from build123d import *

# Parameters (mm, degrees)
SKETCH1_R           = 4.25
BOSS_EXTRUDE1_DEPTH = 9.6
BOSS_EXTRUDE2_DEPTH = 3.3
SKETCH3_OUTSIDE_W   = 42.178
SKETCH3_OUTSIDE_H   = 40.63
SKETCH3_OUTSIDE_R   = 4.25
CUT_EXTRUDE4_DEPTH  = 3.3
CUT_EXTRUDE4_TAPER  = 75
SKETCH5_OUTSIDE_W   = 42.178
SKETCH5_OUTSIDE_H   = 40.63
SKETCH5_OUTSIDE_R   = 4.25
CUT_EXTRUDE5_DEPTH  = 3.3
CUT_EXTRUDE5_TAPER  = 75
SKETCH6_R           = 2.9
BOSS_EXTRUDE3_DEPTH = 3
SKETCH7_R           = 3.95
BOSS_EXTRUDE4_DEPTH = 7.5
SKETCH8_R           = 1.5
CUT_EXTRUDE6_DEPTH  = 24.4
SKETCH9_R           = 2.25
CUT_EXTRUDE7_DEPTH  = 10
FILLET1_R           = 0.5
SKETCH10_R          = 1.5
CUT_EXTRUDE8_DEPTH  = 6.0000001
CHAMFER1_SIZE       = 1


with BuildPart() as part:
    # Sketch1 → Boss-Extrude1 (new body)
    with BuildSketch(Plane(origin=(0, 0, 0), x_dir=(1, 0, 0), z_dir=(0, 1, 0))):
        Circle(SKETCH1_R)
    extrude(amount=BOSS_EXTRUDE1_DEPTH)

    # Sketch2 → Boss-Extrude2 (add)
    with BuildSketch(Plane.XZ):
        Polygon((-2.886751346, 5), (-5.773502692, 0), (-2.886751346, -5), (2.886751346, -5), (5.773502692, 0), (2.886751346, 5), align=None)
    extrude(amount=BOSS_EXTRUDE2_DEPTH)

    # Sketch3 outside → Cut-Extrude4 (cut)
    with BuildSketch(Plane.XZ.offset(3.3)):
        Rectangle(SKETCH3_OUTSIDE_W, SKETCH3_OUTSIDE_H)
        Circle(SKETCH3_OUTSIDE_R, mode=Mode.SUBTRACT)
    extrude(amount=-CUT_EXTRUDE4_DEPTH, taper=CUT_EXTRUDE4_TAPER, mode=Mode.SUBTRACT)

    # Sketch5 outside → Cut-Extrude5 (cut)
    with BuildSketch(Plane(origin=(0, 0, 0), x_dir=(1, 0, 0), z_dir=(0, 1, 0))):
        Rectangle(SKETCH5_OUTSIDE_W, SKETCH5_OUTSIDE_H)
        Circle(SKETCH5_OUTSIDE_R, mode=Mode.SUBTRACT)
    extrude(amount=-CUT_EXTRUDE5_DEPTH, taper=CUT_EXTRUDE5_TAPER, mode=Mode.SUBTRACT)

    # Sketch6 → Boss-Extrude3 (add)
    with BuildSketch(Plane.XZ.offset(3.3)):
        Circle(SKETCH6_R)
    extrude(amount=BOSS_EXTRUDE3_DEPTH)

    # Sketch7 → Boss-Extrude4 (add)
    with BuildSketch(Plane.XZ.offset(6.3)):
        Circle(SKETCH7_R)
    extrude(amount=BOSS_EXTRUDE4_DEPTH)

    # Sketch8 → Cut-Extrude6 (cut, through all)
    with BuildSketch(Plane.XZ.offset(13.8)):
        Circle(SKETCH8_R)
    extrude(amount=-CUT_EXTRUDE6_DEPTH, mode=Mode.SUBTRACT)

    # Sketch9 → Cut-Extrude7 (cut)
    with BuildSketch(Plane.XZ.offset(13.8)):
        Circle(SKETCH9_R)
    extrude(amount=-CUT_EXTRUDE7_DEPTH, mode=Mode.SUBTRACT)

    # Fillet1
    fillet1_edges = [part.edges().sort_by_distance(p)[0] for p in [
        (-4.25, 0, 0),
        (-2.9, -3.3, 0),
        (-2.9, -6.3, 0),
    ]]
    fillet(fillet1_edges, radius=FILLET1_R)

    # Sketch10 → Cut-Extrude8 (cut, through all)
    with BuildSketch(Plane.XY):
        with Locations((0, 5.6)):
            Circle(SKETCH10_R)
    extrude(amount=-CUT_EXTRUDE8_DEPTH, mode=Mode.SUBTRACT)

    # Chamfer1
    chamfer1_edges = [part.edges().sort_by_distance(p)[0] for p in [
        (-2.25, -13.8, 0),
    ]]
    chamfer(chamfer1_edges, length=CHAMFER1_SIZE)


solid = part.part
Source: CAD feature listing. Evaluate the final solid. Frame: model axes, mm. A direction names the side the tool comes from. Round coordinates to 2 decimals unless told otherwise and drop trailing zeros. Write each loop counter-clockwise with the first axis right and the second up, starting at its lowest first coordinate (ties: lowest second). Pieces come first, ordered by that corner, then holes. Notation, with made-up numbers: M -33,8 L -15,8 A30 ccw -15,41 Z; hole C -33.75,63.25 d6. An arc over 180 degrees is marked long. One line per item, written item: value. Start each with the question number.
Item 1: Pin query (flat end, axial travel): pin 1 (1 mm diameter, centred on y = 5, z = 0, fed in from +X); pin 2 (1.5 mm diameter, centred on x = -1, z = 1, fed in from -Y); pin 3 (5 mm diameter, centred on x = 0, z = 0.5, fed in from -Y). Return the tip coordinate at first contact, or that it passes through.
Item 2: Ray query, L1, parallel to Y at x = -1.5, z = 3.5; L2, parallel to X at y = 5.5, z = 0; L3, parallel to Y at x = 0, z = -1.75. Return the intervals inside material, ascending. Write a range as from..to.
Item 3: Section query B-B (x = 0). State how many separate pieces and enclosed holes the cut face has, plus the area to 3 significant figures.
Item 4: Section query A-A (y = 7.75). Return the cut outline in (x, z).
Item 5: Mould query, pull axis Z, two halves, no side actions, for faces 5 (the cylindrical face through (-0.29, -8.36, 2.23)), 6 (the cylindrical face through (-0.195, 2.806, 1.487)), 7 (the flat face through (-2, -3.3, 3)), 8 (the flat face through (4.31, -1.63, -2.535)). Classes: pulls with the +Z half, pulls with the -Z half, needs draft (parallel to the pull), parting line crosses it, or undercut.
Item 6: Section query C-C (y = -9.5). Return the cut outline in (x, z).
Item 7: Set-up query: faces 1 (the flat face through (2, -6.3, 3)), 2 (the cylindrical face through (1.43, 6.05, -2.57)), 3 (the cylindrical face through (1.96, 4.93, 3.77)), 4 (the flat face through (0, -2, 5)). Return all of +Z, -Z, +X, -X, +Y, -Y with unobstructed straight access to the full face (end or side cutting, diameter ignored); none if empty.
Result set:
1. pin 1: stops at x = 4.25
1. pin 2: stops at y = -3.8
1. pin 3: stops at y = -13.55
2. L1: y = -13.8..-6.3, -3.3..9.6
2. L2: x = -4.25..-1.5, 1.5..4.25
2. L3: y = -3.8..4.1, 7.1..9.6
3. separate pieces: 3
3. enclosed holes: 0
3. area: 96.8 mm²
4. outline: C 0,0 d8.5; hole C 0,0 d3
5. face 5: undercut
5. face 6: undercut
5. face 7: needs draft
5. face 8: pulls with the -Z half
6. outline: C 0,0 d7.9; hole C 0,0 d4.5
7. face 1: none
7. face 2: -Z
7. face 3: +Y
7. face 4: +Z, +X, -X, +Y, -Y
